For this review, take the finished solid that the model builds, in its own axes (mm). Face numbers are marked on the shaded views. A direction names the side the tool comes from. Give positions to 0.01 mm unless a question says otherwise; leave off trailing zeros. Order: outer loops, then holes, each group sorted by start corner. A loop starts at its lowest first (then second) coordinate and runs counter-clockwise, first axis right, second up. Notation, with made-up numbers: M -33,65 L 21,65 A14 ccw 21,71 Z; hole C 53,-17 d11. An arc over 180 degrees is marked long. Use CSV: the item, a comma, the result in double quotes. Start each with the question number.
(1) Draft analysis for pull direction Y (two halves, no side actions). For the marked faces 3, 4 and 5, state which applies: pulls with the +Y half, pulls with the -Y half, needs draft (parallel to the pull), parting line crosses it, or undercut.
(2) Wall thickness on L1, parallel to Y at x = 20, z = 5.5; L2, parallel to X at y = 19, z = 3.75; L3, parallel to Y at x = -14.5, z = 15.25: over which ranges is each line inside the solid? List them lowest first. Write a range as from..to.
(3) Consider section D-D (z = 18.5). Write out the cut boundary in (x, y).
(4) Consider section B-B (y = 4). Write out the cut boundary in (x, z).
(5) Tool access review of the marked faces 1 and 2: name each direction out of +Z, -Z, +X, -X, +Y, -Y from which nothing blocks a thin tool from reaching the whole face with its end or side.
(6) Clearance check with flat-ended pins moving along their axes: P1, Ø3.5, axis at y = -43.5, z = 9.5, coming from the +X side; P2, Ø5, axis at x = 0.5, y = 12.5, coming from the +Z side; P3, Ø2.5, axis at x = -38.5, z = 11.5, coming from the +Y side; P4, Ø3.5, axis at x = -38.5, y = 6, coming from the +Z side. State where each tip first meets the part, or that it passes through.
(7) Consider section C-C (x = -13). Write out the cut boundary in (y, z).
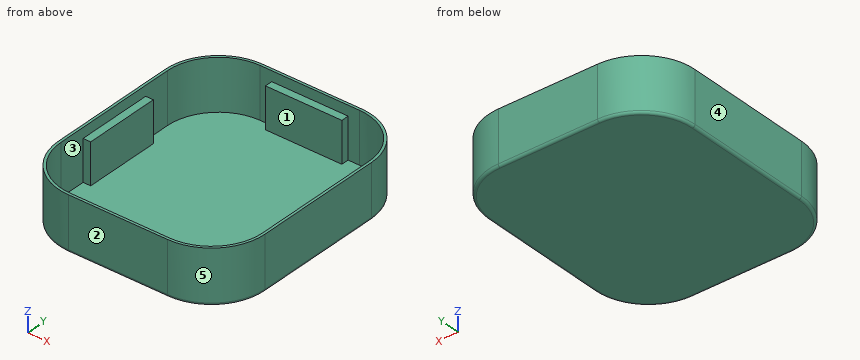
```python
from build123d import *

# Parameters (mm, degrees)
PAD_DEPTH     = 20
THICKNESS_T   = 1
SKETCH001_W   = 3
SKETCH001_H   = 30
SKETCH001_W_2 = 30
SKETCH001_H_2 = 3
PAD001_DEPTH  = 16
PAD002_DEPTH  = 16


with BuildPart() as part:
    # Sketch → Pad (new body)
    with BuildSketch(Plane.XY):
        with BuildLine():
            Line((-19.5, 45.5), (19.5, 45.5))
            ThreePointArc((39.5, 25.5), (33.642136, 39.642136), (19.5, 45.5))
            Line((39.5, 25.5), (39.5, -25.5))
            ThreePointArc((19.5, -45.5), (33.642136, -39.642136), (39.5, -25.5))
            Line((19.5, -45.5), (-19.5, -45.5))
            ThreePointArc((-39.5, -25.5), (-33.642136, -39.642136), (-19.5, -45.5))
            Line((-39.5, -25.5), (-39.5, 25.5))
            ThreePointArc((-19.5, 45.5), (-33.642136, 39.642136), (-39.5, 25.5))
        make_face()
    extrude(amount=PAD_DEPTH)

    # Thickness
    thickness_openings = [part.faces().sort_by_distance(p)[0] for p in [
        (0, 0, 20),
    ]]
    offset(amount=THICKNESS_T, openings=thickness_openings)

    # Sketch001 (on Face9 of Thickness) → Pad001 (join)
    with BuildSketch(Plane.XY):
        with Locations((-38, 0)):
            Rectangle(SKETCH001_W, SKETCH001_H)
        with Locations((38, 0)):
            Rectangle(SKETCH001_W, SKETCH001_H)
        with Locations((0, -44)):
            Rectangle(SKETCH001_W_2, SKETCH001_H_2)
        with Locations((0, 44)):
            Rectangle(SKETCH001_W_2, SKETCH001_H_2)
    extrude(amount=PAD001_DEPTH)

    # Sketch001 (on Face9 of Thickness) → Pad002 (join)
    with BuildSketch(Plane.XY):
        with Locations((-38, 0)):
            Rectangle(SKETCH001_W, SKETCH001_H)
        with Locations((38, 0)):
            Rectangle(SKETCH001_W, SKETCH001_H)
        with Locations((0, -44)):
            Rectangle(SKETCH001_W_2, SKETCH001_H_2)
        with Locations((0, 44)):
            Rectangle(SKETCH001_W_2, SKETCH001_H_2)
    extrude(amount=PAD002_DEPTH)


solid = part.part
```
Check result:
1,face 3,"undercut"
1,face 4,"needs draft"
1,face 5,"pulls with the -Y half"
2,L1,"y = -46.49..-45.49, 45.49..46.49"
2,L2,"x = -40.5..-39.5, 39.5..40.5"
2,L3,"y = -46.5..-42.5, 42.5..46.5"
3,outline,"M -40.5,-25.5 A21 ccw -19.5,-46.5 L 19.5,-46.5 A21 ccw 40.5,-25.5 L 40.5,25.5 A21 ccw 19.5,46.5 L -19.5,46.5 A21 ccw -40.5,25.5 Z; hole M -39.5,-25.5 A20 ccw -19.5,-45.5 L 19.5,-45.5 A20 ccw 39.5,-25.5 L 39.5,25.5 A20 ccw 19.5,45.5 L -19.5,45.5 A20 ccw -39.5,25.5 Z"
4,outline,"M -40.5,0 A1 ccw -39.5,-1 L 39.5,-1 A1 ccw 40.5,0 L 40.5,20 L 39.5,20 L 39.5,16 L 36.5,16 L 36.5,0 L -36.5,0 L -36.5,16 L -39.5,16 L -39.5,20 L -40.5,20 Z"
5,face 1,"+Z"
5,face 2,"+Z, -Z, +X, -X, -Y"
6,P1,"stops at x = 32.8"
6,P2,"stops at z = 0"
6,P3,"stops at y = 36.72"
6,P4,"stops at z = 20"
7,outline,"M -46.5,0 A1 ccw -45.5,-1 L 45.5,-1 A1 ccw 46.5,0 L 46.5,20 L 45.5,20 L 45.5,16 L 42.5,16 L 42.5,0 L -42.5,0 L -42.5,16 L -45.5,16 L -45.5,20 L -46.5,20 Z"
